from build123d import *

# Parameters (mm, degrees)
SKETCH1_W           = 37.7
SKETCH1_H           = 25
BOSS_EXTRUDE1_DEPTH = 0.3
CUT_EXTRUDE1_REACH  = 24.62
SKETCH2_W           = 15
SKETCH2_H           = 6


with BuildPart() as part:
    # Sketch1 → Boss-Extrude1 (new body)
    with BuildSketch(Plane.XY):
        Rectangle(SKETCH1_W, SKETCH1_H)
    extrude(amount=BOSS_EXTRUDE1_DEPTH)

    # Sketch2 → Cut-Extrude1 (cut, up to next)
    with BuildSketch(Plane.XY.offset(0.3), mode=Mode.PRIVATE) as cut_extrude1_sk1:
        with Locations((0, -11.7)):
            Rectangle(SKETCH2_W, SKETCH2_H)
    cut_extrude1_tool1 = extrude(cut_extrude1_sk1.sketch, amount=-CUT_EXTRUDE1_REACH, mode=Mode.PRIVATE) & part.part
    add(cut_extrude1_tool1.solids().sort_by_distance((0, -11.7, 0.3))[0], mode=Mode.SUBTRACT)


solid = part.part
Work out the finished part from the listing and answer in its coordinate system (mm). Round coordinates to 2 decimals unless told otherwise and drop trailing zeros. Write each loop counter-clockwise with the first axis right and the second up, starting at its lowest first coordinate (ties: lowest second). Pieces come first, ordered by that corner, then holes. Notation, with made-up numbers: M 81.5,12.5 L 140.5,12.5 A23 cw 140.5,32.5 Z; hole C 11,-31.75 d11. An arc over 180 degrees is marked long. Use a Markdown table: item, result.
1) The part is cut by section B-B on y = -10.75. Give the vertices of the cut face in (x, z).
Taken from the geometry:
| item | result |
|---|---|
| outline | M -18.85,0 L -7.5,0 L -7.5,0.3 L -18.85,0.3 Z; M 7.5,0 L 18.85,0 L 18.85,0.3 L 7.5,0.3 Z |
2) The part is cut by section A-A on z = 0.2. Give the vertices of the cut face in (x, y).
Taken from the geometry:
| item | result |
|---|---|
| outline | M -18.85,-12.5 L -7.5,-12.5 L -7.5,-8.7 L 7.5,-8.7 L 7.5,-12.5 L 18.85,-12.5 L 18.85,12.5 L -18.85,12.5 Z |
3) Consider line 1 (Y direction, x = 7, z = 0.2). Determine where the line is inside the solid, lowest interval first. Write a range as [from, to].
Taken from the geometry:
| item | result |
|---|---|
| line 1 | y = [-8.7, 12.5] |
4) The part is cut by section C-C on x = 4.5. Give the vertices of the cut face in (y, z), plus the area to 3 significant figures.
Taken from the geometry:
| item | result |
|---|---|
| outline | M -8.7,0 L 12.5,0 L 12.5,0.3 L -8.7,0.3 Z |
| area | 6.36 mm2 |
